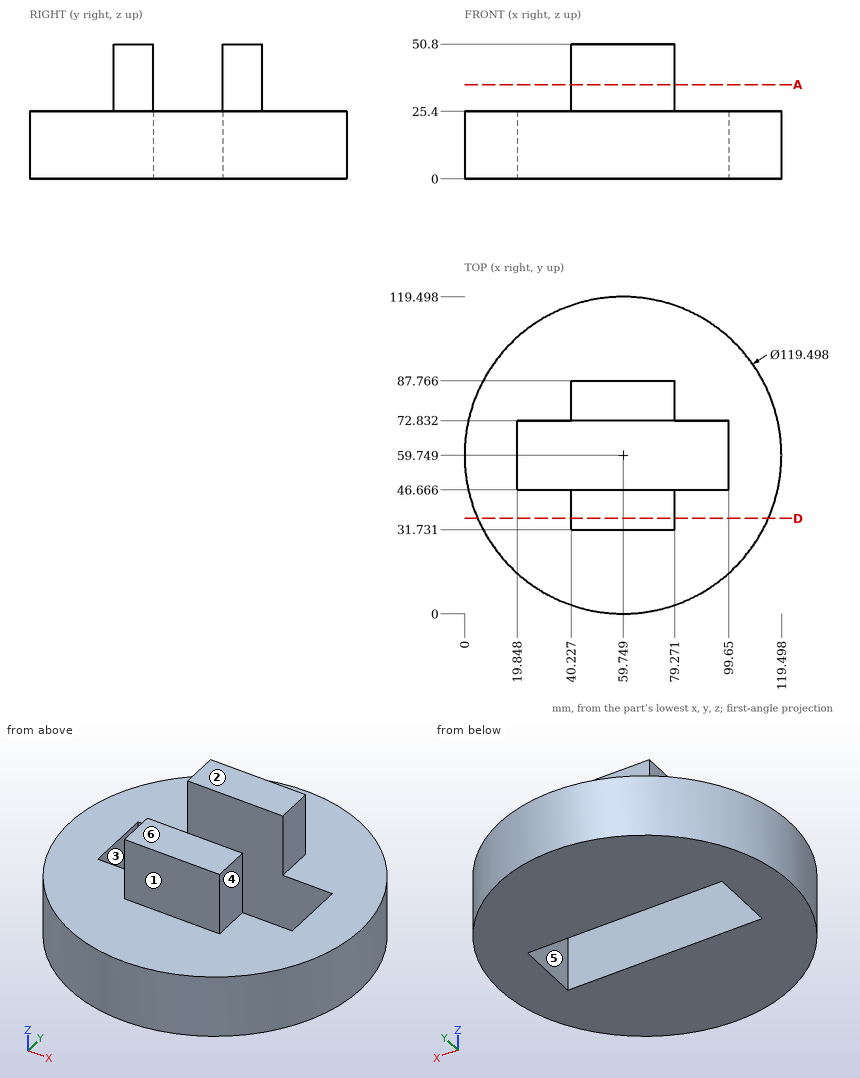
Study the drawing (mm; zero at the part's minimum x, y, z) and answer. A direction names the side the tool comes from. Give positions to 0.01 mm unless a question says otherwise; leave off trailing zeros. Loops run counter-clockwise (first coordinate to the right, second up) from the corner with the lowest first, then second, coordinate; pieces in that order, holes last. Notation, with made-up numbers: (40, 73) - (49, 73) arc R6 cw to (49, 77) - close; hole circle Ø4 at (63, 2). An arc over 180 degrees is marked (long way). Return JSON: item names as keys, results as strings. Group by question number.
1. Given pin 1 Ø4 at (x, z) = (31, 13) entering from -Y; pin 2 Ø15 at (x, z) = (70, 16) entering from -Y; pin 3 Ø7.5 at (y, z) = (41.5, 43) entering from -X, each flat-ended and moving along its own axis, determine where each tip first touches the part or whether it passes through.
2. Find section A-A (z = 35.5). Write down the section's boundary in (x, y) (1 decimal).
3. Determine the mould class of the marked faces 1, 2 and 3 for opening direction Y: pulls with the +Y half, pulls with the -Y half, needs draft (parallel to the pull), parting line crosses it, or undercut.
4. Find section D-D (y = 36). Write down the section's boundary in (x, z) (1 decimal).
5. Straight lines are drawn through the part: line 1 (Y direction, x = 75, z = 48) (1 decimal); line 2 (Z direction, x = 26, y = 89); line 3 (X direction, y = 44, z = 35.5). For each, find the intervals that lie inside material, in ascending order. Write a range as [from, to].
6. Which of the six approach directions +Z, -Z, +X, -X, +Y, -Y give full straight-line access (tool end or side, diameter ignored) to the marked faces 4, 5 and 6?
Verdict:
{
 "1": {"pin 1": "stops at y = 6.32", "pin 2": "stops at y = 0.06", "pin 3": "stops at x = 40.23"},
 "2": {"outline": "(40.2, 31.7) - (79.3, 31.7) - (79.3, 46.7) - (40.2, 46.7) - close; (40.2, 72.8) - (79.3, 72.8) - (79.3, 87.8) - (40.2, 87.8) - close"},
 "3": {"face 1": "pulls with the -Y half", "face 2": "needs draft", "face 3": "undercut"},
 "4": {"outline": "(4.9, 0) - (114.6, 0) - (114.6, 25.4) - (79.3, 25.4) - (79.3, 50.8) - (40.2, 50.8) - (40.2, 25.4) - (4.9, 25.4) - close"},
 "5": {"line 1": "y = [31.7, 46.7], [72.8, 87.8]", "line 2": "z = [0, 25.4]", "line 3": "x = [40.23, 79.27]"},
 "6": {"face 4": "+Z, +X, +Y, -Y", "face 5": "+Z, -Z", "face 6": "+Z, +X, -X, +Y, -Y"}
}
